```python
from build123d import *

# Parameters (mm, degrees)
SKETCH_W         = 21
SKETCH_H         = 21
SKETCH_W_2       = 15
SKETCH_H_2       = 15
PAD_DEPTH        = 2.5
SKETCH001_W      = 21
SKETCH001_H      = 21
SKETCH001_R      = 2.075
PAD001_DEPTH     = 4
SKETCH002_W      = 21
SKETCH002_H      = 21
SKETCH002_W_2    = 14.5
SKETCH002_H_2    = 14.5
PAD002_DEPTH     = 2.3
CHAMFER_SIZE     = 3
SKETCH003_R      = 0.75
POCKET_DEPTH     = 8.801
CHAMFER001_SIZE2 = 3.999
CHAMFER001_SIZE  = 1.8


with BuildPart() as part:
    # Sketch → Pad (new body)
    with BuildSketch(Plane.XY):
        Rectangle(SKETCH_W, SKETCH_H)
        Rectangle(SKETCH_W_2, SKETCH_H_2, mode=Mode.SUBTRACT)
    extrude(amount=PAD_DEPTH)

    # Sketch001 (on Face9 of Pad) → Pad001 (join)
    with BuildSketch(Plane(origin=(0, 0, 0), x_dir=(1, 0, 0), z_dir=(0, 0, -1))):
        Rectangle(SKETCH001_W, SKETCH001_H)
        Circle(SKETCH001_R, mode=Mode.SUBTRACT)
    extrude(amount=PAD001_DEPTH)

    # Sketch002 (on Face5 of Pad001) → Pad002 (join)
    with BuildSketch(Plane.XY.offset(2.5)):
        Rectangle(SKETCH002_W, SKETCH002_H)
        Rectangle(SKETCH002_W_2, SKETCH002_H_2, mode=Mode.SUBTRACT)
    extrude(amount=PAD002_DEPTH)

    # Chamfer
    chamfer_edges = [part.edges().sort_by_distance(p)[0] for p in [
        (-10.5, -10.5, -2),
        (10.5, -10.5, -2),
        (10.5, 10.5, -2),
        (-10.5, 10.5, -2),
    ]]
    chamfer(chamfer_edges, length=CHAMFER_SIZE)

    # Sketch003 (on Face8 of Chamfer) → Pocket (cut, through all)
    with BuildSketch(Plane(origin=(0, 0, -4), x_dir=(1, 0, 0), z_dir=(0, 0, -1))):
        with Locations((4, 2.85)):
            Circle(SKETCH003_R)
        with Locations((-2.9, 5)):
            Circle(SKETCH003_R)
    extrude(amount=-POCKET_DEPTH, mode=Mode.SUBTRACT)

    # Chamfer001
    chamfer001_edges = [part.edges().sort_by_distance(p)[0] for p in [
        (3.25, -2.85, -4),
        (-3.65, -5, -4),
    ]]
    chamfer001_side = part.faces().sort_by_distance((0, -10.203015, -4))[0]
    chamfer(chamfer001_edges, length=CHAMFER001_SIZE, length2=CHAMFER001_SIZE2, reference=chamfer001_side)


solid = part.part
```
Geometry: final body of the model. Coordinates: model frame, mm. A direction names the side the tool comes from. Round coordinates to 2 decimals unless told otherwise and drop trailing zeros. Order: outer loops, then holes, each group sorted by start corner. A loop starts at its lowest first (then second) coordinate and runs counter-clockwise, first axis right, second up. Notation, with made-up numbers: M 29,-23.5 L 63,-23.5 A13 cw 63,-10.5 Z; hole C 12.25,88 d3. An arc over 180 degrees is marked long. One line per item, written item: value.
(1) Pull-direction query (Z, two-part tool) for faces 4 (the flat face through (-8, -2, 4.8)), 5 (the flat face through (7.5, 0, 1)), 6 (the cylindrical face through (-0.45, 2.026, -1.972)), 7 (the flat face through (-2.5, -0.1, -4)); classes: pulls with the +Z half, pulls with the -Z half, needs draft (parallel to the pull), parting line crosses it, or undercut.
Result sheet:
face 4: pulls with the +Z half
face 5: undercut
face 6: needs draft
face 7: pulls with the -Z half
(2) Cut plane D-D (z = -1). Return the cut outline in (x, y) (3 decimals).
Result sheet:
outline: M -10.5,-7.5 L -7.5,-10.5 L 7.5,-10.5 L 10.5,-7.5 L 10.5,7.5 L 7.5,10.5 L -7.5,10.5 L -10.5,7.5 Z; hole C -2.9,-5 d2.399; hole C 0,0 d4.15; hole C 4,-2.85 d2.399
(3) Pin query (flat end, axial travel): P1, Ø5.5, axis at x = 0, y = 0, coming from the +Z side; P2, Ø2, axis at x = 4, y = -2.85, coming from the -Z side. Return the tip coordinate at first contact, or that it passes through.
Result sheet:
P1: z = 0
P2: z = -0.56
(4) Cut plane C-C (z = 0.75). Return the cut outline in (x, y), and give its area (3 significant figures).
Result sheet:
outline: M -10.5,-7.5 L -7.5,-10.5 L 7.5,-10.5 L 10.5,-7.5 L 10.5,7.5 L 7.5,10.5 L -7.5,10.5 L -10.5,7.5 Z; hole M -7.5,-7.5 L 7.5,-7.5 L 7.5,7.5 L -7.5,7.5 Z
area: 198 mm2
(5) Cut plane B-B (y = 0). Return the cut outline in (x, z) (3 decimals).
Result sheet:
outline: M -10.5,-4 L -2.075,-4 L -2.075,0 L -7.5,0 L -7.5,2.5 L -7.25,2.5 L -7.25,4.8 L -10.5,4.8 Z; M 2.075,-4 L 10.5,-4 L 10.5,4.8 L 7.25,4.8 L 7.25,2.5 L 7.5,2.5 L 7.5,0 L 2.075,0 Z
(6) Reachability of faces 1 (the flat face through (9, -9, 0)), 2 (the flat face through (0, -7.25, 4)), 3 (the flat face through (0, 7.5, 1)) from +Z, -Z, +X, -X, +Y, -Y: full face, straight path, thin tool, end or side. Return the list, or none.
Result sheet:
face 1: +Z, -Z, +X, -Y
face 2: +Z
face 3: none
(7) Line query: probe 1 along X at (y, z) = (0, -0.95) (3 decimals); probe 2 along Y at (x, z) = (-2.9, 0.05); probe 3 along X at (y, z) = (3.25, 4). Output: solid intervals per line, ascending. Write a range as [from, to].
Result sheet:
probe 1: [-10.5, -2.075], [2.075, 10.5]
probe 2: [-10.5, -7.5], [7.5, 10.5]
probe 3: [-10.5, -7.25], [7.25, 10.5]
